Geometry check sheet. Reference: the model listing, model coordinates, mm. A direction names the side the tool comes from. Round coordinates to 2 decimals unless told otherwise and drop trailing zeros. Order: outer loops, then holes, each group sorted by start corner. A loop starts at its lowest first (then second) coordinate and runs counter-clockwise, first axis right, second up. Notation, with made-up numbers: (74, 44) - (109, 44) arc R19 cw to (109, 65) - close; hole circle Ø3 at (-15.75, 66.5). An arc over 180 degrees is marked (long way). Return JSON: item names as keys, results as strings. Group by question number.
Q1. Draft check along Y on faces 1 (the flat face through (106, -52.386, 119)), 2 (the cylindrical face through (-28.727, 36.368, 118.874)), 3 (the flat face through (-2, -125, 105)), 4 (the flat face through (-2, 125, 105)). Enter one of: pulls with the +Y half, pulls with the -Y half, needs draft (parallel to the pull), parting line crosses it, or undercut.
Q2. Tool access check on faces 5 (the flat face through (117.636, 66, 119)), 6 (the flat face through (106, 52.386, 119)), 7 (the flat face through (-2, -110, 1)), 8 (the flat face through (94.636, 66, 119)), 9 (the cylindrical face through (3.465, -73.759, 118.874)). Record the directions out of +Z, -Z, +X, -X, +Y, -Y that give a thin tool (end or side, any length) a straight path to the whole face; none if there is none.
Q3. Sectioned sample at C-C, the plane y = -89. Record the cut outline in (x, z), then the cut area to 3 significant figures.
Q4. Sectioned sample at A-A, the plane x = 105. Record the cut outline in (y, z).
Q5. Material ranges on line 1 along Y through (x, z) = (-105, 62.5); line 2 along Z through (x, y) = (118.5, 107.5), recorded low to high.
Q6. Sectioned sample at D-D, the plane x = 10. Record the cut outline in (y, z).
Q7. Gauge pin test, flat ends, axial feed: pin 1 Ø20 at (y, z) = (-68.5, 119.5) entering from +X; pin 2 Ø9 at (x, z) = (105.5, 122.5) entering from +Y; pin 3 Ø9 at (y, z) = (-62.5, 123.5) entering from -X; pin 4 Ø8 at (x, z) = (-8.5, -31.5) entering from +Y. Record the tip position at first contact, or that the pin passes through.
Q8. Sectioned sample at B-B, the plane z = 70. Record the cut outline in (x, y), then the cut area to 3 significant figures.
```python
from build123d import *

# Parameters (mm, degrees)
F0_W     = 300
F0_H     = 200
F1_DEPTH = 110
F2_W     = 300
F2_H     = 250
F3_DEPTH = 10
F4_R     = 25
F4_W     = 23
F4_H     = 28
F5_DEPTH = 18


with BuildPart() as f1:
    # F0 (on Front) → F1 (new body, symmetric)
    with BuildSketch(Plane.XZ):
        Rectangle(F0_W, F0_H)
    extrude(amount=F1_DEPTH, both=True)

    # F2 (on face) → F3 (join)
    with BuildSketch(Plane.XY.offset(100)):
        Rectangle(F2_W, F2_H)
    extrude(amount=F3_DEPTH)

    # F4 (on face) → F5 (join)
    with BuildSketch(Plane.XY.offset(110)):
        with Locations((-107.0935577154, 58.547321707)):
            Circle(F4_R)
        with Locations((-40.2627661824, 58.547321707)):
            Circle(F4_R)
        with Locations((23.3044344932, 58.547321707)):
            Circle(F4_R)
        with Locations((-107.0935577154, -58.547321707)):
            Circle(F4_R)
        with Locations((-40.2627661824, -58.547321707)):
            Circle(F4_R)
        with Locations((23.3044344932, -58.547321707)):
            Circle(F4_R)
        with Locations((106.136246562, 66.3863844573)):
            Rectangle(F4_W, F4_H)
        with Locations((106.136246562, -66.3863844573)):
            Rectangle(F4_W, F4_H)
    extrude(amount=F5_DEPTH)


solid = f1.part
```
Reply:
{
 "1": {"face 1": "undercut", "face 2": "undercut", "face 3": "pulls with the -Y half", "face 4": "pulls with the +Y half"},
 "2": {"face 5": "+Z, +X, +Y, -Y", "face 6": "+Z, +X", "face 7": "-Z, +X, -X, -Y", "face 8": "+Z, +Y, -Y", "face 9": "+Z"},
 "3": {"outline": "(-150, -100) - (150, -100) - (150, 110) - (-150, 110) - close", "area": "63,000 mm^2"},
 "4": {"outline": "(-125, 100) - (-110, 100) - (-110, -100) - (110, -100) - (110, 100) - (125, 100) - (125, 110) - (80.39, 110) - (80.39, 128) - (52.39, 128) - (52.39, 110) - (-52.39, 110) - (-52.39, 128) - (-80.39, 128) - (-80.39, 110) - (-125, 110) - close"},
 "5": {"line 1": "-110 to 110", "line 2": "-100 to 110"},
 "6": {"outline": "(-125, 100) - (-110, 100) - (-110, -100) - (110, -100) - (110, 100) - (125, 100) - (125, 110) - (79.71, 110) - (79.71, 128) - (37.38, 128) - (37.38, 110) - (-37.38, 110) - (-37.38, 128) - (-79.71, 128) - (-79.71, 110) - (-125, 110) - close"},
 "7": {"pin 1": "x = 150", "pin 2": "y = 80.39", "pin 3": "x = -132.09", "pin 4": "y = 110"},
 "8": {"outline": "(-150, -110) - (150, -110) - (150, 110) - (-150, 110) - close", "area": "66,000 mm^2"}
}
